Read the model definition and answer for the solid it produces. Units are mm, in the model's axes. A direction names the side the tool comes from. Give positions to 0.01 mm unless a question says otherwise; leave off trailing zeros. Write each loop counter-clockwise with the first axis right and the second up, starting at its lowest first coordinate (ties: lowest second). Pieces come first, ordered by that corner, then holes. Notation, with made-up numbers: (41, 18) - (98, 18) arc R9 ccw to (98, 24) - close; hole circle Ø7 at (78, 65.25). An arc over 180 degrees is marked (long way). Use CSV: the item, a comma, the result in double quotes. Start each with the question number.
from build123d import *

# Parameters (mm, degrees)
SKETCH2_R          = 8.5725
EXTRUDE1_DEPTH     = 13.97
EXTRUDE1_DRAFT     = 1.5
CHAMFER1_SIZE      = 1.062566667
CHAMFER1_SIZE2     = 1.091513185
EXTRUDE2_DEPTH     = 5.08
SKETCH12_OUTSIDE_W = 110.834
SKETCH12_OUTSIDE_H = 113.196
SKETCH12_OUTSIDE_R = 8.763
CUT_EXTRUDE6_DEPTH = 24.349152203
CUT_EXTRUDE6_DRAFT = -60
SKETCH13_OUTSIDE_W = 97.25
SKETCH13_OUTSIDE_H = 99.612
SKETCH13_OUTSIDE_R = 8.763
CUT_EXTRUDE7_DEPTH = 20.42784879
CUT_EXTRUDE7_DRAFT = -60
SKETCH16_R         = 3.175
CUT_EXTRUDE8_DEPTH = 24.349152203


with BuildPart() as part:
    # Sketch2 → Extrude1 (with draft: the straight prism first)
    with BuildSketch(Plane(origin=(9.525, 0, 0), x_dir=(0, 0, -1), z_dir=(1, 0, 0))):
        Circle(SKETCH2_R)
    extrude(amount=-EXTRUDE1_DEPTH)
    # Extrude1: the draft: its side faces are tilted about the plane it starts from
    extrude1_sides = [part.faces().sort_by_distance(p)[0] for p in [
        (2.54, 0, 8.5725),
    ]]
    draft(extrude1_sides, Plane(origin=(9.525, 0, 0), x_dir=(0, 0, -1), z_dir=(1, 0, 0)), EXTRUDE1_DRAFT)

    # Chamfer1
    chamfer1_edges = [part.edges().sort_by_distance(p)[0] for p in [
        (9.525, 0, 8.5725),
    ]]
    chamfer1_side = [part.faces().sort_by_distance(p)[0] for p in [
        (2.54, 0, 8.755408662),
    ]]
    chamfer(chamfer1_edges, length=CHAMFER1_SIZE, length2=CHAMFER1_SIZE2, reference=chamfer1_side[0])

    # Sketch5 → Extrude2 (add)
    with BuildSketch(Plane.ZY.offset(4.445)):
        Polygon((0, 10.118640818), (-8.763, 5.059320409), (-8.763, -5.059320409), (0, -10.118640818), (8.763, -5.059320409), (8.763, 5.059320409), align=None)
    extrude(amount=EXTRUDE2_DEPTH)


with BuildPart() as cut_extrude6_tool:
    # Sketch12 outside → Cut-Extrude6 (with draft: the straight prism first)
    with BuildSketch(Plane.ZY.offset(9.525)):
        Rectangle(SKETCH12_OUTSIDE_W, SKETCH12_OUTSIDE_H)
        Circle(SKETCH12_OUTSIDE_R, mode=Mode.SUBTRACT)
    extrude(amount=-CUT_EXTRUDE6_DEPTH)
    # Cut-Extrude6: the draft: its side faces are tilted about the plane it starts from
    cut_extrude6_sides = [cut_extrude6_tool.faces().sort_by_distance(p)[0] for p in [
        (2.649576101, -56.598, 0),
        (2.649576101, 0, 55.417),
        (2.649576101, 56.598, 0),
        (2.649576101, 0, -55.417),
        (2.649576101, 0, -8.763),
    ]]
    draft(cut_extrude6_sides, Plane.ZY.offset(9.525), CUT_EXTRUDE6_DRAFT)


with BuildPart() as part_1:
    add(part.part)

    # Cut-Extrude6: cut by cut_extrude6_tool
    add(cut_extrude6_tool.part, mode=Mode.SUBTRACT)


with BuildPart() as cut_extrude7_tool:
    # Sketch13 outside → Cut-Extrude7 (with draft: the straight prism first)
    with BuildSketch(Plane(origin=(-4.445, 0, 0), x_dir=(0, 0, -1), z_dir=(1, 0, 0))):
        Rectangle(SKETCH13_OUTSIDE_W, SKETCH13_OUTSIDE_H)
        Circle(SKETCH13_OUTSIDE_R, mode=Mode.SUBTRACT)
    extrude(amount=-CUT_EXTRUDE7_DEPTH)
    # Cut-Extrude7: the draft: its side faces are tilted about the plane it starts from
    cut_extrude7_sides = [cut_extrude7_tool.faces().sort_by_distance(p)[0] for p in [
        (-14.658924395, -49.806, 0),
        (-14.658924395, 0, -48.625),
        (-14.658924395, 49.806, 0),
        (-14.658924395, 0, 48.625),
        (-14.658924395, 0, 8.763),
    ]]
    draft(cut_extrude7_sides, Plane(origin=(-4.445, 0, 0), x_dir=(0, 0, -1), z_dir=(1, 0, 0)), CUT_EXTRUDE7_DRAFT)


with BuildPart() as part_2:
    add(part_1.part)

    # Cut-Extrude7: cut by cut_extrude7_tool
    add(cut_extrude7_tool.part, mode=Mode.SUBTRACT)

    # Sketch16 → Cut-Extrude8 (cut, through all)
    with BuildSketch(Plane.ZY.offset(9.525)):
        Circle(SKETCH16_R)
    extrude(amount=-CUT_EXTRUDE8_DEPTH, mode=Mode.SUBTRACT)


solid = part_2.part
(1) Which of the six approach directions +Z, -Z, +X, -X, +Y, -Y give full straight-line access (tool end or side, diameter ignored) to faces 4 (the face through (-7, 0, -8.763)), 5 (the face through (-9.338, -9.086, -0.022)), 6 (the face through (-6.949, -7.624, 4.32))?
(2) Given P1, Ø4, axis at x = 4.5, z = -7, coming from the +Y side; P2, Ø2.5, axis at x = -6, y = -2, coming from the -Z side; P3, Ø3, axis at x = -2.5, z = 7, coming from the -Y side, each flat-ended and moving along its own axis, determine where each tip first touches the part or whether it passes through.
(3) For a pull along Z with two mould halves and no side action, classify faces 1 (the face through (2.1, -8.56, 1.9)), 2 (the face through (-6.949, 7.554, 4.443)), 3 (the face through (-0.13, -3.1, -0.69)) as pulls with the +Z half, pulls with the -Z half, needs draft (parallel to the pull), parting line crosses it, or undercut.
(4) The part is cut by section C-C on x = 5.25. Write down the section's boundary in (y, z) (3 decimals), plus the area to 3 significant figures.
(5) The part is cut by section B-B on x = -3.5. Write down the section's boundary in (y, z) (3 decimals), plus the area to 3 significant figures.
(6) Consider probe 1 along Y at (x, z) = (1.5, 0) (3 decimals); probe 2 along Y at (x, z) = (0.5, 2.75); probe 3 along Z at (x, y) = (-4, -2). Determine where each line is inside the solid, lowest interval first.
(7) The part is cut by section A-A on x = -7. Write down the section's boundary in (y, z) (3 decimals), plus the area to 3 significant figures.
Reported:
1,face 4,"-Z, -X, +Y, -Y"
1,face 5,"-X, -Y"
1,face 6,"+Z, -X, -Y"
2,P1,"y = 7.13"
2,P2,"z = -8.76"
2,P3,"y = -6.98"
3,face 1,"parting line crosses it"
3,face 2,"pulls with the +Z half"
3,face 3,"undercut"
4,outline,"circle Ø17.369 at (0, 0); hole circle Ø6.35 at (0, 0)"
4,area,"205 mm²"
5,outline,"circle Ø17.827 at (0, 0); hole circle Ø6.35 at (0, 0)"
5,area,"218 mm²"
6,probe 1,"-8.783 to -3.175, 3.175 to 8.783"
6,probe 2,"-8.37 to -1.59, 1.59 to 8.37"
6,probe 3,"-8.7 to -2.47, 2.47 to 8.7"
7,outline,"(-10.119, 0) - (-5.059, -8.763) - (5.059, -8.763) - (10.119, 0) - (5.059, 8.763) - (-5.059, 8.763) - close; hole circle Ø6.35 at (0, 0)"
7,area,"234 mm²"
